Autodesk Fusion 360 part; units mm, degrees
sketch "Sketch1" plane through (0, 0, 0) normal (0, 0, 1) x (1, 0, 0)
  line L0 (-9.0933, 15.75) -> (-18.1865, 0)
  line L1 (-18.1865, 0) -> (-9.0933, -15.75)
  line L2 (-9.0933, -15.75) -> (9.0933, -15.75)
  line L3 (9.0933, -15.75) -> (18.1865, 0)
  line L4 (18.1865, 0) -> (9.0933, 15.75)
  line L5 (9.0933, 15.75) -> (-9.0933, 15.75)
  dimension "d8" = 31.5
extrude "Extrude1" add sketch "Sketch1" along normal blind 56.1
sketch "Sketch3" plane through (0, 0, 56.1) normal (0, 0, 1) x (-1, 0, 0)
  line L0 (-9.0933, -15.75) -> (9.0933, -15.75)
  line L1 (9.0933, -15.75) -> (18.1865, 0)
  line L2 (18.1865, 0) -> (9.0933, 15.75)
  line L3 (9.0933, 15.75) -> (-9.0933, 15.75)
  line L4 (-9.0933, 15.75) -> (-18.1865, 0)
  line L5 (-18.1865, 0) -> (-9.0933, -15.75)
hole "Hole1" at (0, 0, 56.1) direction (0, 0, -1) diameter 18 end through all
sketch "Sketch4" plane through (0, 0, 0) normal (0, 0, -1) x (1, 0, 0)
  circle A0 centre (0, 0) radius 9
  line L0 (-9.0933, -15.75) -> (9.0933, -15.75)
  line L1 (9.0933, -15.75) -> (18.1865, 0)
  line L2 (18.1865, 0) -> (9.0933, 15.75)
  line L3 (9.0933, 15.75) -> (-9.0933, 15.75)
  line L4 (-9.0933, 15.75) -> (-18.1865, 0)
  line L5 (-18.1865, 0) -> (-9.0933, -15.75)
  circle A1 centre (0, 0) radius 9
  circle A2 centre (0, 0) radius 5
  dimension "d12" = 10
extrude "Extrude3" add sketch "Sketch4" against normal blind 2.1 contours A0 A1
sketch "Sketch5" plane through (0, 0, 56.1) normal (0, 0, 1) x (-1, 0, 0)
  circle A0 centre (0, 0) radius 9
  line L0 (-9.0933, -15.75) -> (9.0933, -15.75)
  line L1 (9.0933, -15.75) -> (18.1865, 0)
  line L2 (18.1865, 0) -> (9.0933, 15.75)
  line L3 (9.0933, 15.75) -> (-9.0933, 15.75)
  line L4 (-9.0933, 15.75) -> (-18.1865, 0)
  line L5 (-18.1865, 0) -> (-9.0933, -15.75)
  line L6 (8.4004, -14.55) -> (16.8009, 0)
  line L7 (16.8009, 0) -> (8.4004, 14.55)
  line L8 (8.4004, 14.55) -> (-8.4004, 14.55)
  line L9 (-8.4004, 14.55) -> (-16.8009, 0)
  line L10 (-16.8009, 0) -> (-8.4004, -14.55)
  line L11 (-8.4004, -14.55) -> (8.4004, -14.55)
  dimension "d15" = 29.1
extrude "Extrude4" add sketch "Sketch5" along normal blind 0.9 contours L0 L1 L2 L3 L4 L5
sketch "Sketch6" plane through (0, 0, 0) normal (0, 0, -1) x (-1, 0, 0)
  line L0 (8.4004, -14.55) -> (-8.4004, -14.55)
  line L1 (-8.4004, -14.55) -> (-16.8009, 0)
  line L2 (-16.8009, 0) -> (-8.4004, 14.55)
  line L3 (-8.4004, 14.55) -> (8.4004, 14.55)
  line L4 (8.4004, 14.55) -> (16.8009, 0)
  line L5 (16.8009, 0) -> (8.4004, -14.55)
  line L6 (-18.1865, 0) -> (-9.0933, -15.75)
  line L7 (-9.0933, -15.75) -> (9.0933, -15.75)
  line L8 (9.0933, -15.75) -> (18.1865, 0)
  line L9 (18.1865, 0) -> (9.0933, 15.75)
  line L10 (9.0933, 15.75) -> (-9.0933, 15.75)
  line L11 (-9.0933, 15.75) -> (-18.1865, 0)
  circle A0 centre (0, 0) radius 7
  circle A1 centre (0, 0) radius 9
  circle A2 centre (0, 0) radius 5
  line L12 (9.0933, 15.75) -> (-9.0933, 15.75)
  line L13 (-9.0933, 15.75) -> (-18.1865, 0)
  line L14 (-18.1865, 0) -> (-9.0933, -15.75)
  line L15 (-9.0933, -15.75) -> (9.0933, -15.75)
  line L16 (9.0933, -15.75) -> (18.1865, 0)
  line L17 (18.1865, 0) -> (9.0933, 15.75)
  dimension "d18" = 14
extrude "Extrude5" add sketch "Sketch6" against normal blind 20.4 contours A1
equation "d8 = 29.1 mm + 2.4 mm"
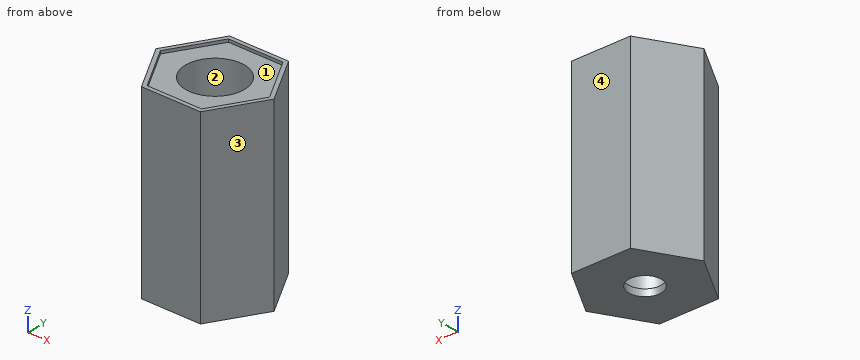
For this review, take the finished solid that the model builds, in its own axes (mm). Face numbers are marked on the shaded views. Coordinates: 2 decimals unless noted, no trailing zeros. Order: outer loops, then holes, each group sorted by start corner. A loop starts at its lowest first (then second) coordinate and runs counter-clockwise, first axis right, second up. Notation, with made-up numbers: (72, 19) - (88, 19) arc R36 cw to (88, 53) - close; hole circle Ø4 at (42.5, 23). An arc over 180 degrees is marked (long way). Use one line per item in the form item = value.
Q1. Consider section C-C (x = 0). Give the boundary of the cut face in (y, z), then the cut area to 3 significant figures.
Checked values:
outline = (-15.75, 0) - (-5, 0) - (-5, 2.1) - (-7, 2.1) - (-7, 20.4) - (-9, 20.4) - (-9, 56.1) - (-14.55, 56.1) - (-14.55, 57) - (-15.75, 57) - close; (5, 0) - (15.75, 0) - (15.75, 57) - (14.55, 57) - (14.55, 56.1) - (9, 56.1) - (9, 20.4) - (7, 20.4) - (7, 2.1) - (5, 2.1) - close
area = 850 mm2
Q2. Consider section B-B (y = -2). Give the boundary of the cut face in (x, z).
Checked values:
outline = (-17.03, 0) - (-4.58, 0) - (-4.58, 2.1) - (-6.71, 2.1) - (-6.71, 20.4) - (-8.77, 20.4) - (-8.77, 56.1) - (-15.65, 56.1) - (-15.65, 57) - (-17.03, 57) - close; (4.58, 0) - (17.03, 0) - (17.03, 57) - (15.65, 57) - (15.65, 56.1) - (8.77, 56.1) - (8.77, 20.4) - (6.71, 20.4) - (6.71, 2.1) - (4.58, 2.1) - close
Q3. Draft analysis for pull direction X (two halves, no side actions). For the marked faces 1, 2, 3 and 4, state which applies: +X half, -X half, draft (parallel to the pull), parting line (faces both ways), or undercut.
Checked values:
face_1 = undercut
face_2 = undercut
face_3 = +X half
face_4 = draft
Q4. Consider section D-D (z = 15.5). Give the boundary of the cut face in (x, y).
Checked values:
outline = (-18.19, 0) - (-9.09, -15.75) - (9.09, -15.75) - (18.19, 0) - (9.09, 15.75) - (-9.09, 15.75) - close; hole circle Ø14 at (0, 0)
Q5. Consider section A-A (z = 34). Give the boundary of the cut face in (x, y), then the cut area to 3 significant figures.
Checked values:
outline = (-18.19, 0) - (-9.09, -15.75) - (9.09, -15.75) - (18.19, 0) - (9.09, 15.75) - (-9.09, 15.75) - close; hole circle Ø18 at (0, 0)
area = 605 mm2
Q6. For P1, Ø1, axis at y = 6, z = 47.5, coming from the +X side; P2, Ø10, axis at y = -4.5, z = 32.5, coming from the +X side; P3, Ø12, axis at y = -12.5, z = 36, coming from the +X side; P4, Ø12.5, axis at x = 0, y = 0, coming from the +Z side, all flat-tipped, find the tip position at first contact; note any pin that passes through.
Checked values:
P1 = 15.01
P2 = 18.19
P3 = 14.43
P4 = 2.1
Q7. For probe 1 along Y at (x, z) = (0, 1); probe 2 along X at (y, z) = (0, 39); probe 3 along Y at (x, z) = (0, 13.25), list the stretches that pass through material, from the lowest coordinate up. Write a range as from..to.
Checked values:
probe_1 = -15.75..-5, 5..15.75
probe_2 = -18.19..-9, 9..18.19
probe_3 = -15.75..-7, 7..15.75
